Autodesk Inventor part; units mm, degrees
ref_plane "Piano iniziale" through (0, 0, 0) normal (0, 0, 1) x (1, 0, 0)
ref_plane "Piano finale" through (0, 0, 620) normal (0, 0, 1) x (1, 0, 0)
ref_plane "YZ Plane" through (0, 0, 0) normal (1, 0, 0) x (0, 1, 0)
ref_plane "Piano iniziale" through (0, 0, 0) normal (0, 0, 1) x (1, 0, 0)
ref_plane "Piano finale" through (0, 0, 620) normal (0, 0, 1) x (1, 0, 0)
sketch "Schizzo" plane through (0, 0, 0) normal (0, 0, 1) x (1, 0, 0)
  line L0 (-20, -16) -> (-20, 16)
  line L1 (-16, 20) -> (16, 20)
  line L2 (20, 16) -> (20, -16)
  line L3 (16, -20) -> (-16, -20)
  arc A0 (-20, -16) -> (-16, -20) centre (-16, -16) ccw
  arc A1 (20, 16) -> (16, 20) centre (16, 16) ccw
  arc A2 (-16, 20) -> (-20, 16) centre (-16, 16) ccw
  arc A3 (16, -20) -> (20, -16) centre (16, -16) ccw
  arc A4 (-16, 18) -> (-18, 16) centre (-16, 16) ccw
  line L4 (-16, 18) -> (16, 18)
  arc A5 (18, 16) -> (16, 18) centre (16, 16) ccw
  line L5 (18, 16) -> (18, -16)
  arc A6 (16, -18) -> (18, -16) centre (16, -16) ccw
  line L6 (16, -18) -> (-16, -18)
  arc A7 (-18, -16) -> (-16, -18) centre (-16, -16) ccw
  line L7 (-18, -16) -> (-18, 16)
  line L8 (0, 29.1598) -> (0, -29.1598) construction
  line L9 (-29.1598, 0) -> (29.1598, 0) construction
  dimension "d7" = 4
  dimension "d9" = 40
  dimension "d11" = 40
  dimension "d12" = 2
  dimension "d15" = 20
  dimension "d16" = 20
extrude "Corpo" add sketch "Schizzo" along normal up to surface (620 mm away) from surface at 0
sketch "Sketch3" plane through (0, 0, 0) normal (0, 0, 1) x (1, 0, 0)
  line L0 (0, 0) -> (10, 0)
ref_plane "Work Plane3" through (0, 0, 0) normal (0, -1, 0) x (1, 0, 0)
sketch "Sketch4" plane through (0, 0, 0) normal (0, -1, 0) x (1, 0, 0)
  line L0 (-2, 0) -> (12, 0)
  line L1 (-2, 620) -> (12, 620)
  dimension "d18" = 620
sketch "Schizzo5" plane through (-20, 16, 0) normal (-1, 0, 0) x (0, 0, 1)
  line L0 (0, -36) -> (620, -36)
  line L1 (0, -32) -> (0, 0)
  point P0 (0, -16)
  point P1 (75, -23.5)
  point P2 (285, -23.5)
  point P3 (390, -23.5)
  point P4 (180, -23.5)
  dimension "d22" = 105
  dimension "d30" = 12.5
  dimension "d31" = 75
  dimension "d32" = 105
  dimension "d33" = 105
hole "Foro1" at (-20, -7.5, 75) at (-20, -7.5, 285) at (-20, -7.5, 390) at (-20, -7.5, 180) direction (1, 0, 0) diameter 10 depth 5 tip angle 118
equation "\"d7\" = G_IR"
equation "\"d9\" = G_W"
equation "\"d11\" = G_H"
equation "\"d12\" = G_T"
equation "\"d15\" = 0.5 * d9"
equation "\"d16\" = 0.5 * d11"
equation "\"d3\" = G_L"
equation "\"G_W\" = 40"
equation "\"G_H\" = 40"
equation "\"G_T\" = 2"
equation "\"G_IR\" = 4"
equation "\"G_L\" = d18"
equation "\"G_OFFSET_START\" = 0"
equation "\"G_OFFSET_END\" = 0"
properties part number "ISO 10799-2 - 40x40x2 - 620" material "Acciaio, Dolce"
CAD build for the part. Positions are in the model's coordinates, mm. A direction names the side the tool comes from. Give positions to 0.01 mm unless a question says otherwise; leave off trailing zeros. Loops run counter-clockwise (first coordinate to the right, second up) from the corner with the lowest first, then second, coordinate; pieces in that order, holes last. Notation, with made-up numbers: M -24,76 L 1,76 A25 ccw 1,109 Z; hole C 22.5,23 d8. An arc over 180 degrees is marked long. Answer in a Markdown table with one row per item. Add a question column.
Item 1: Band-saw the part on B-B on z = 191. Give the cut face in (x, y).
Item 2: Band-saw the part on C-C on z = 285. Give the cut face in (x, y).
Item 3: Band-saw the part on A-A on x = -10. Give the cut face in (y, z).
Item 4: Probe probe 1 along Z at (x, y) = (-19, -7.5); probe 2 along X at (y, z) = (-5, 421). List the from-to ranges inside material, lowest first.
Item 5: Tool access for faces 5 (the face through (20, 0, 306)), 6 (the face through (-18, 0, 306)), 7 (the face through (-18.99, -9, 289.77)): list every direction of +Z, -Z, +X, -X, +Y, -Y with a clear straight run to the whole face (end or side of a thin tool).
Item 6: Mould opens along X. For faces 1 (the face through (-2, -19, 620)), 2 (the face through (-20, 0, 306)), 3 (the face through (18, 0, 306)), 4 (the face through (0, 18, 306)) say: +X half, -X half, draft (parallel to the pull), parting line (faces both ways), or undercut.
Reply:
| question | item | result |
|---|---|---|
| 1 | outline | M -20,-16 A4 ccw -16,-20 L 16,-20 A4 ccw 20,-16 L 20,16 A4 ccw 16,20 L -16,20 A4 ccw -20,16 Z; hole M -18,-16 A2 ccw -16,-18 L 16,-18 A2 ccw 18,-16 L 18,16 A2 ccw 16,18 L -16,18 A2 ccw -18,16 Z |
| 2 | outline | M -20,-16 A4 ccw -16,-20 L 16,-20 A4 ccw 20,-16 L 20,16 A4 ccw 16,20 L -16,20 A4 ccw -20,16 L -20,-2.5 L -18,-2.5 L -18,16 A2 cw -16,18 L 16,18 A2 cw 18,16 L 18,-16 A2 cw 16,-18 L -16,-18 A2 cw -18,-16 L -18,-12.5 L -20,-12.5 Z |
| 3 | outline | M -20,0 L -18,0 L -18,620 L -20,620 Z; M 18,0 L 20,0 L 20,620 L 18,620 Z |
| 4 | probe 1 | z = 0 to 70, 80 to 175, 185 to 280, 290 to 385, 395 to 620 |
| 4 | probe 2 | x = -20 to -18, 18 to 20 |
| 5 | face 5 | +Z, -Z, +X, +Y, -Y |
| 5 | face 6 | +Z, -Z |
| 5 | face 7 | -X |
| 6 | face 1 | draft |
| 6 | face 2 | -X half |
| 6 | face 3 | undercut |
| 6 | face 4 | undercut |
